The listing builds one solid part. Answer for the finished solid, in the listing's coordinates (mm). A direction names the side the tool comes from. Coordinates: 2 decimals unless noted, no trailing zeros. Order: outer loops, then holes, each group sorted by start corner. A loop starts at its lowest first (then second) coordinate and runs counter-clockwise, first axis right, second up. Notation, with made-up numbers: (55, 64) - (65, 64) arc R18 cw to (65, 82) - close; hole circle Ø4 at (6, -11). An arc over 180 degrees is marked (long way). Use a Markdown table: item, result. Add a question column.
Item 1: Find the intervals of material crossed by line 1 along Z through (x, y) = (25.5, 0.7); line 2 along X through (y, z) = (1.6, -10.75); line 3 along X through (y, z) = (1.15, -17.5), in increasing order.
Item 2: The part is cut by section A-A, the plane x = 3. Give the vertices of the cut face in (y, z).
Item 3: For faces 1 (the cylindrical face through (8, 1, -15)), 2 (the flat face through (82, 1, 0)), determine the directions among +Z, -Z, +X, -X, +Y, -Y from which every point of the face is accessible in a straight line to the end or side of a thin tool.
Item 4: The part is cut by section B-B, the plane y = 0.8. Give the vertices of the cut face in (x, z).
Item 5: A flat-ended cylindrical pin translates along its axis: P1, Ø1.8, axis at x = 3, z = -3, coming from the -Y side. Find the tip coordinate at first contact, or state that the pin passes through.
Item 6: The part is cut by section C-C, the plane x = 55. Give the vertices of the cut face in (y, z), then the cut area to 3 significant figures.
Item 7: The part is cut by section D-D, the plane z = -13.75. Give the vertices of the cut face in (x, y), then the cut area to 3 significant figures.
from build123d import *

# Parameters (mm, degrees)
SKETCH1_W           = 166.159725664
SKETCH1_H           = 20
SKETCH1_R           = 1.5
SKETCH1_W_2         = 154.159725664
SKETCH1_H_2         = 12
BOSS_EXTRUDE1_DEPTH = 3
CUT_EXTRUDE1_DEPTH  = 168.38594455
FILLET1_R           = 5


with BuildPart() as part:
    # Sketch1 → Boss-Extrude1 (new body)
    with BuildSketch(Plane(origin=(0, 0, 0), x_dir=(1, 0, 0), z_dir=(0, 1, 0))):
        with Locations((83.079862832, 10)):
            Rectangle(SKETCH1_W, SKETCH1_H)
        with Locations(Location((3, 17, 0), (0, 0, 270))):
            Circle(SKETCH1_R, mode=Mode.SUBTRACT)
        with Locations(Location((3, 3, 0), (0, 0, 90))):
            Circle(SKETCH1_R, mode=Mode.SUBTRACT)
        with Locations(Location((163.159725664, 3, 0), (0, 0, 270))):
            Circle(SKETCH1_R, mode=Mode.SUBTRACT)
        with Locations(Location((163.159725664, 17, 0), (0, 0, 90))):
            Circle(SKETCH1_R, mode=Mode.SUBTRACT)
        with Locations((83.079862832, 10)):
            Rectangle(SKETCH1_W_2, SKETCH1_H_2, mode=Mode.SUBTRACT)
    extrude(amount=BOSS_EXTRUDE1_DEPTH)

    # Sketch2 → Cut-Extrude1 (cut, through all)
    with BuildSketch(Plane(origin=(0, 3, 0), x_dir=(1, 0, 0), z_dir=(0, 1, 0))):
        Polygon((147.159725664, 17), (147.159725664, 16), (160.159725664, 16), (160.159725664, 4), (147.159725664, 4), (147.159725664, 3), (161.159725664, 3), (161.159725664, 17), align=None)
    extrude(amount=-CUT_EXTRUDE1_DEPTH, mode=Mode.SUBTRACT)

    # Fillet1
    # the kernel refuses this fillet: 5 mm, written as the material it adds along each edge
    with BuildSketch(Plane(origin=(161.159725664, 3, -17), x_dir=(0, 0, 1), z_dir=(0, -1, 0)), Plane(origin=(161.159725664, 3, -3), x_dir=(-1, 0, 0), z_dir=(0, -1, 0)), Plane(origin=(6, 0, -16), x_dir=(0, 0, 1), z_dir=(0, 1, 0))) as fillet1_piece_1:
        with BuildLine():
            CenterArc((FILLET1_R, FILLET1_R), FILLET1_R, 180, 90)
            Line((0, FILLET1_R), (-FILLET1_R * 0.02, FILLET1_R))
            Line((-FILLET1_R * 0.02, FILLET1_R), (-FILLET1_R * 0.02, -FILLET1_R * 0.02))
            Line((-FILLET1_R * 0.02, -FILLET1_R * 0.02), (FILLET1_R, -FILLET1_R * 0.02))
            Line((FILLET1_R, -FILLET1_R * 0.02), (FILLET1_R, 0))
        make_face()
    extrude(amount=3)
    with BuildSketch(Plane(origin=(147.159725664, 3, -17), x_dir=(1, 0, 0), z_dir=(0, -1, 0))) as fillet1_piece_2:
        with BuildLine():
            CenterArc((3, 5), FILLET1_R, 233.130102354, 36.869897646)
            Line((0, 1), (-0.06, 0.92))
            ThreePointArc((-0.06, 0.92), (-0.1, 0.5), (-0.1, 0))
            Line((-0.1, 0), (0, -0.1))
            Line((0, -0.1), (3, -0.1))
            Line((3, -0.1), (3, 0))
        make_face()
    extrude(amount=3)
    with BuildSketch(Plane(origin=(147.159725664, 3, -3), x_dir=(0, 0, -1), z_dir=(0, -1, 0))) as fillet1_piece_3:
        with BuildLine():
            CenterArc((5, 3), FILLET1_R, 180, 36.869897646)
            Line((0, 3), (-0.1, 3))
            Line((-0.1, 3), (-0.1, 0))
            Line((-0.1, 0), (0, -0.1))
            ThreePointArc((0, -0.1), (0.5, -0.1), (0.92, -0.06))
            Line((0.92, -0.06), (1, 0))
        make_face()
    extrude(amount=3)
    with BuildSketch(Plane(origin=(6, 0, -4), x_dir=(0, 0, -1), z_dir=(0, 1, 0))) as fillet1_piece_4:
        with BuildLine():
            CenterArc((FILLET1_R, -FILLET1_R), FILLET1_R, 90, 90)
            Line((0, -FILLET1_R), (-FILLET1_R * 0.02, -FILLET1_R))
            Line((-FILLET1_R * 0.02, -FILLET1_R), (-FILLET1_R * 0.02, FILLET1_R * 0.02))
            Line((-FILLET1_R * 0.02, FILLET1_R * 0.02), (FILLET1_R, FILLET1_R * 0.02))
            Line((FILLET1_R, FILLET1_R * 0.02), (FILLET1_R, 0))
        make_face()
    extrude(amount=3)


solid = part.part
Solution:
| question | item | result |
|---|---|---|
| 1 | line 1 | z = -20 to -16, -4 to 0 |
| 1 | line 2 | x = 0 to 6, 161.16 to 166.16 |
| 1 | line 3 | x = 0 to 1.59, 4.41 to 161.75, 164.57 to 166.16 |
| 2 | outline | (0, -20) - (3, -20) - (3, -18.5) - (0, -18.5) - close; (0, -15.5) - (3, -15.5) - (3, -4.5) - (0, -4.5) - close; (0, -1.5) - (3, -1.5) - (3, 0) - (0, 0) - close |
| 3 | face 1 | +Y, -Y |
| 3 | face 2 | +Z, +X, -X, +Y, -Y |
| 4 | outline | (0, -20) - (166.16, -20) - (166.16, 0) - (0, 0) - close; hole circle Ø3 at (3, -17); hole circle Ø3 at (3, -3); hole (6, -11) arc R5 ccw to (11, -16) - (147.16, -16) arc R5 ccw to (150.16, -17) - (156.16, -17) arc R5 ccw to (161.16, -12) - (161.16, -8) arc R5 ccw to (156.16, -3) - (150.16, -3) arc R5 ccw to (147.16, -4) - (11, -4) arc R5 ccw to (6, -9) - close; hole circle Ø3 at (163.16, -17); hole circle Ø3 at (163.16, -3) |
| 5 | P1 | passes through |
| 6 | outline | (0, -20) - (3, -20) - (3, -16) - (0, -16) - close; (0, -4) - (3, -4) - (3, 0) - (0, 0) - close |
| 6 | area | 24.0 mm2 |
| 7 | outline | (0, 0) - (6.82, 0) - (6.82, 3) - (0, 3) - close; (160.84, 0) - (166.16, 0) - (166.16, 3) - (160.84, 3) - close |
| 7 | area | 36.4 mm2 |
